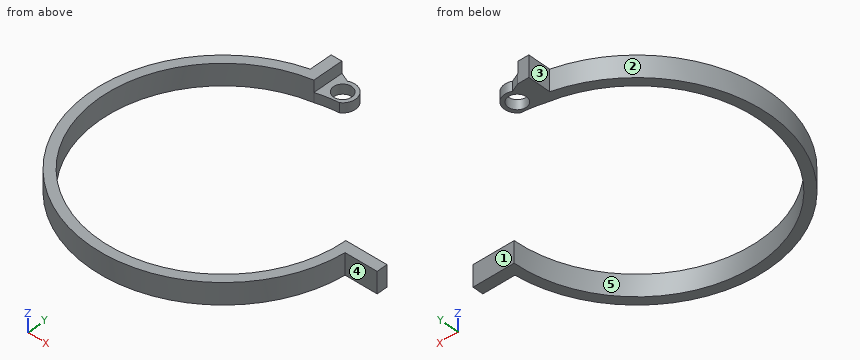
```python
from build123d import *

# Parameters (mm, degrees)
SKETCH_R        = 4.25
PAD_DEPTH       = 10
POCKET_DEPTH    = 5.5
POCKET001_DEPTH = 5


with BuildPart() as part:
    # Sketch → Pad (new body)
    with BuildSketch(Plane.XY):
        with BuildLine():
            ThreePointArc((-9.98477, 56.626446), (-36.960288, -44.047555), (57.5, 0))
            Line((57.5, 0), (76.798058, 0))
            Line((76.798058, 0), (76.798058, -5))
            Line((76.798058, -5), (61.798058, -5))
            ThreePointArc((-14.984756, 60.161924), (-40.117208, -47.271657), (61.798058, -5))
            Line((-14.984756, 60.161924), (-14.984756, 70.757167))
            Line((-14.984756, 70.757167), (5.015244, 70.757167))
            Line((5.015244, 70.757167), (5.015244, 58.757167))
            ThreePointArc((5.015244, 58.757167), (-2.560203, 58.222895), (-9.98477, 56.626446))
        make_face()
        with Locations((-2.984756, 63.626448)):
            Circle(SKETCH_R, mode=Mode.SUBTRACT)
    extrude(amount=PAD_DEPTH)

    # Sketch001 (on Face12 of Pad) → Pocket (cut)
    with BuildSketch(Plane.XY.offset(10)):
        with BuildLine():
            ThreePointArc((5.1, 58.499907), (-2.531657, 57.967199), (-10.00931, 56.351442))
            Line((-10.00931, 56.351442), (-10.00931, 70.999907))
            Line((-10.00931, 70.999907), (5.1, 70.999907))
            Line((5.1, 70.999907), (5.1, 58.499907))
        make_face()
    extrude(amount=-POCKET_DEPTH, mode=Mode.SUBTRACT)

    # Sketch002 (on Face6 of Pocket) → Pocket001 (cut)
    with BuildSketch(Plane.XY.offset(4.5)):
        with BuildLine():
            ThreePointArc((-1, 57.993146), (2.515586, 66.011846), (-5.713792, 69.001199))
            Line((-5.713792, 69.001199), (-11.5, 71.493146))
            Line((-11.5, 71.493146), (6, 71.493146))
            Line((6, 71.493146), (6, 57.993146))
            Line((6, 57.993146), (-1, 57.993146))
        make_face()
    extrude(amount=-POCKET001_DEPTH, mode=Mode.SUBTRACT)


solid = part.part
```
Here's how the part is built. I have some questions about the finished solid (model axes, mm). Face numbers are marked on the shaded views. A direction names the side the tool comes from. Give positions to 0.01 mm unless a question says otherwise; leave off trailing zeros. Loops run counter-clockwise (first coordinate to the right, second up) from the corner with the lowest first, then second, coordinate; pieces in that order, holes last. Notation, with made-up numbers: M 85.25,-15.5 L 134.25,-15.5 A15 cw 134.25,5.5 Z; hole C 15,56 d8. An arc over 180 degrees is marked long. Use one line per item in the form item = value. Start each with the question number.
Q1. If we section it at B-B (z = 1.75): Write out the boundary of the cut face in (x, y).
Q2. Thinking about a two-plate mould opening in X: for the marked faces 3, 4 and 5, which applies, +X half, -X half, draft (parallel to the pull), parting line (faces both ways), or undercut?
Q3. Will these pins go through, and if not, where does the flat tip stop? pin 1 Ø1 at (x, z) = (8, 6.5) entering from -Y; pin 2 Ø4 at (x, y) = (-6.5, 63) entering from +Z; pin 3 Ø1 at (x, z) = (57, 1) entering from -Y.
Q4. If we section it at C-C (y = 17.5): Write out the boundary of the cut face in (x, z), then the cut area to 3 significant figures.
Q5. If we section it at A-A (x = -3): Write out the boundary of the cut face in (y, z), then the cut area to 3 significant figures.
Q6. If we section it at D-D (x = 30.5): Write out the boundary of the cut face in (y, z), then the cut area to 3 significant figures.
Q7. I need wall thicknesses on line 1 along X through (y, z) = (-2, 1); line 2 along Y through (x, z) = (0, 3.5); line 3 along X through (y, z) = (-10, 4.5). Which ranges of each line are inside material? Lowest first, please.
Q8. Which directions (+Z, -Z, +X, -X, +Y, -Y) give clear straight access to the entire face, cutting with the end or side of a thin tool? Please do the marked faces 1 and 2.
Taken from the geometry:
q1.outline = M -14.98,60.16 A62 ccw long 61.8,-5 L 76.8,-5 L 76.8,0 L 57.5,0 A57.5 cw long -9.98,56.63 A53.76 cw 0.14,58.54 A6 ccw -5.71,69 L -9.79,70.76 L -14.98,70.76 Z; hole C -2.98,63.63 d8.5
q2.face_3 = -X half
q2.face_4 = draft
q2.face_5 = undercut
q3.pin_1 = -61.54
q3.pin_2 = 4.5
q3.pin_3 = -25.53
q4.outline = M -59.48,0 L -54.77,0 L -54.77,10 L -59.48,10 Z
q4.area = 47.1 mm^2
q5.outline = M -61.93,0 L -57.42,0 L -57.42,10 L -61.93,10 Z; M 58.16,0 L 59.38,0 L 59.38,4.5 L 58.16,4.5 Z; M 67.88,0 L 69.65,0 L 69.65,4.5 L 67.88,4.5 Z
q5.area = 58.5 mm^2
q6.outline = M -53.98,0 L -48.74,0 L -48.74,10 L -53.98,10 Z
q6.area = 52.3 mm^2
q7.line_1 = -61.97 to -57.47, 57.47 to 76.8
q7.line_2 = -62 to -57.5, 58.52 to 60.6, 66.65 to 68.85
q7.line_3 = -61.19 to -56.62, 56.62 to 61.19
q8.face_1 = +Z, -Z, +X, +Y
q8.face_2 = +Z, -Z
